from build123d import *

# Parameters (mm, degrees)
SKETCH_1_R      = 2.5
EXTRUDE_1_DEPTH = 1.6
SKETCH_2_W      = 15
SKETCH_2_H      = 18
EXTRUDE_2_DEPTH = 10
SKETCH_3_W      = 10
SKETCH_3_H      = 6.85
SKETCH_3_W_2    = 14.15
SKETCH_3_H_2    = 8.85
SKETCH_3_W_3    = 14
SKETCH_3_H_3    = 9
EXTRUDE_3_DEPTH = 5
SKETCH_1_3_R    = 2.5
SKETCH_1_3_R_2  = 1.5
EXTRUDE_4_DEPTH = 1.6


with BuildPart() as part:
    # Sketch 1 → Extrude 1 (new body)
    with BuildSketch(Plane(origin=(0, 0, 0), x_dir=(1, 0, 0), z_dir=(0, 1, 0))):
        with BuildLine():
            Line((-35, 17.5), (-35, -17.5))
            ThreePointArc((-35, -17.5), (-33.535533906, -21.035533906), (-30, -22.5))
            Line((-30, -22.5), (30, -22.5))
            ThreePointArc((30, -22.5), (33.535533906, -21.035533906), (35, -17.5))
            Line((35, -17.5), (35, 17.5))
            ThreePointArc((35, 17.5), (33.535533906, 21.035533906), (30, 22.5))
            Line((30, 22.5), (-30, 22.5))
            ThreePointArc((-30, 22.5), (-33.535533906, 21.035533906), (-35, 17.5))
        make_face()
        with Locations(Location((30.4, -17.95, 0), (0, 0, 270))):
            Circle(SKETCH_1_R, mode=Mode.SUBTRACT)
        with Locations(Location((30.4, 17.95, 0), (0, 0, 270))):
            Circle(SKETCH_1_R, mode=Mode.SUBTRACT)
        with Locations(Location((-30.4, -17.95, 0), (0, 0, 270))):
            Circle(SKETCH_1_R, mode=Mode.SUBTRACT)
        with Locations(Location((-30.4, 17.95, 0), (0, 0, 270))):
            Circle(SKETCH_1_R, mode=Mode.SUBTRACT)
    extrude(amount=EXTRUDE_1_DEPTH)

    # Sketch 2 → Extrude 2 (add)
    with BuildSketch(Plane(origin=(0, 4.6, 0), x_dir=(1, 0, 0), z_dir=(0, 1, 0))):
        with Locations((-30.75023032, 0)):
            Rectangle(SKETCH_2_W, SKETCH_2_H)
    extrude(amount=-EXTRUDE_2_DEPTH)

    # Sketch 3 → Extrude 3 (add)
    with BuildSketch(Plane.XZ):
        with Locations((-21.9, -18.875)):
            Rectangle(SKETCH_3_W, SKETCH_3_H)
        with Locations((-10.4, -18.875)):
            Rectangle(SKETCH_3_W, SKETCH_3_H)
        with Locations((2.675, -17.875)):
            Rectangle(SKETCH_3_W_2, SKETCH_3_H_2)
        with Locations((18.825, -17.875)):
            Rectangle(SKETCH_3_W_2, SKETCH_3_H_2)
        with Locations((-13.6, 17.8)):
            Rectangle(SKETCH_3_W_3, SKETCH_3_H_3)
        with Locations((2.4, 17.8)):
            Rectangle(SKETCH_3_W_3, SKETCH_3_H_3)
        with Locations((18.4, 17.8)):
            Rectangle(SKETCH_3_W_3, SKETCH_3_H_3)
    extrude(amount=EXTRUDE_3_DEPTH)

    # Sketch 1_3 → Extrude 4 (add)
    # profile 1 of 4: a face of its own
    with BuildSketch(Plane(origin=(0, 0, 0), x_dir=(1, 0, 0), z_dir=(0, 1, 0))):
        with Locations((-30.4, -17.95)):
            Circle(SKETCH_1_3_R)
        with Locations(Location((-30.4, -17.95, 0), (0, 0, 270))):
            Circle(SKETCH_1_3_R_2, mode=Mode.SUBTRACT)
    # profile 2 of 4: a face of its own
    with BuildSketch(Plane(origin=(0, 0, 0), x_dir=(1, 0, 0), z_dir=(0, 1, 0))):
        with Locations((-30.4, 17.95)):
            Circle(SKETCH_1_3_R)
        with Locations(Location((-30.4, 17.95, 0), (0, 0, 270))):
            Circle(SKETCH_1_3_R_2, mode=Mode.SUBTRACT)
    # profile 3 of 4: a face of its own
    with BuildSketch(Plane(origin=(0, 0, 0), x_dir=(1, 0, 0), z_dir=(0, 1, 0))):
        with Locations((30.4, 17.95)):
            Circle(SKETCH_1_3_R)
        with Locations(Location((30.4, 17.95, 0), (0, 0, 270))):
            Circle(SKETCH_1_3_R_2, mode=Mode.SUBTRACT)
    # profile 4 of 4: a face of its own
    with BuildSketch(Plane(origin=(0, 0, 0), x_dir=(1, 0, 0), z_dir=(0, 1, 0))):
        with Locations((30.4, -17.95)):
            Circle(SKETCH_1_3_R)
        with Locations(Location((30.4, -17.95, 0), (0, 0, 270))):
            Circle(SKETCH_1_3_R_2, mode=Mode.SUBTRACT)
    extrude(amount=EXTRUDE_4_DEPTH)


solid = part.part
Source: CAD feature listing. Evaluate the final solid. Frame: model axes, mm. A direction names the side the tool comes from. Round coordinates to 2 decimals unless told otherwise and drop trailing zeros. Order: outer loops, then holes, each group sorted by start corner. A loop starts at its lowest first (then second) coordinate and runs counter-clockwise, first axis right, second up. Notation, with made-up numbers: (11, 55.5) - (69, 55.5) arc R36 cw to (69, 91.5) - close; hole circle Ø5 at (43.25, 0.5). An arc over 180 degrees is marked (long way). Use a Markdown table: item, result. Add a question column.
1. Section query C-C (z = 5). Return the cut outline in (x, y), then the cut area to 3 significant figures.
2. Set-up query: faces 1 (the flat face through (-10, -2, -15.45)), 2 (the flat face through (-22, -2, -22.3)), 3 (the flat face through (9.4, -2, 18)). Return all of +Z, -Z, +X, -X, +Y, -Y with unobstructed straight access to the full face (end or side cutting, diameter ignored); none if empty.
3. Section query A-A (y = -4). Give the number of separate pieces and of enclosed holes in the cut face, then the cut area to 3 significant figures.
4. Line query: probe 1 along X at (y, z) = (0.6, -17.95); probe 2 along Z at (x, y) = (5.5, -0.25); probe 3 along X at (y, z) = (-0.25, -15). Output: solid intervals per line, ascending.
5. Mould query, pull axis X, two halves, no side actions, for faces 4 (the flat face through (-23.25, -3, 0)), 5 (the cylindrical face through (-31.73, 0.79, -17.26)), 6 (the flat face through (-10, -5, -19)). Classes: +X half, -X half, draft (parallel to the pull), parting line (faces both ways), or undercut.
6. First-contact query: pin 1 (1.5 mm diameter, centred on y = -3, z = -19.5, fed in from +X); pin 2 (1.5 mm diameter, centred on x = -14, z = 6, fed in from +Y); pin 3 (1 mm diameter, centred on x = 19.5, y = -3, fed in from +Z). Flat tips, straight axial feed; report the tip coordinate or a pass-through.
7. Section query D-D (x = 0.5). Return the cut outline in (y, z).
8. Section query B-B (x = -19). Return the cut outline in (y, z).
Derived:
| question | item | result |
|---|---|---|
| 1 | outline | (-38.25, -5.4) - (-23.25, -5.4) - (-23.25, 0) - (35, 0) - (35, 1.6) - (-23.25, 1.6) - (-23.25, 4.6) - (-38.25, 4.6) - close |
| 1 | area | 243 mm2 |
| 2 | face 1 | -X, -Y |
| 2 | face 2 | -Z, +X, -X, -Y |
| 2 | face 3 | +Z, -Y |
| 3 | separate pieces | 8 |
| 3 | enclosed holes | 0 |
| 3 | area | 1,040 mm2 |
| 4 | probe 1 | -34.98 to -31.9, -28.9 to 28.9, 31.9 to 34.98 |
| 4 | probe 2 | -22.3 to -13.45, 13.3 to 22.3 |
| 4 | probe 3 | -4.4 to 9.75, 11.75 to 25.9 |
| 5 | face 4 | +X half |
| 5 | face 5 | undercut |
| 5 | face 6 | draft |
| 6 | pin 1 | x = 25.9 |
| 6 | pin 2 | y = 1.6 |
| 6 | pin 3 | z = 22.3 |
| 7 | outline | (-5, -22.3) - (0, -22.3) - (0, -22.5) - (1.6, -22.5) - (1.6, 22.5) - (0, 22.5) - (0, 22.3) - (-5, 22.3) - (-5, 13.3) - (0, 13.3) - (0, -13.45) - (-5, -13.45) - close |
| 8 | outline | (-5, -22.3) - (0, -22.3) - (0, -22.5) - (1.6, -22.5) - (1.6, 22.5) - (0, 22.5) - (0, 22.3) - (-5, 22.3) - (-5, 13.3) - (0, 13.3) - (0, -15.45) - (-5, -15.45) - close |
